```python
from build123d import *

# Parameters (mm, degrees)
F0_W      = 16
F0_H      = 16
F1_DEPTH  = 16
F2_R      = 2.54
F2_R_2    = 0.083649
F3_DEPTH  = 1.27
F3_FACE_R = 0.083649
F4_DEPTH  = 1.27
F5_R      = 2.54
F6_DEPTH  = 1.27
F7_DEPTH  = 1.27
F8_R      = 1.905
F8_R_2    = 1.900447
F9_DEPTH  = 1.27
F10_R     = 1.905
F11_DEPTH = 1.27
F12_R     = 1.872316
F12_R_2   = 1.905
F14_DEPTH = 1.27


with BuildPart() as f1:
    # F0 (on Front) → F1 (new body)
    with BuildSketch(Plane.XZ):
        with Locations((30.6324, 48.480009)):
            Rectangle(F0_W, F0_H)
    extrude(amount=-F1_DEPTH)

    # F2 (on face) → F3 (cut)
    with BuildSketch(Plane.XZ):
        with Locations((30.6324, 48.39636)):
            Circle(F2_R)
        with Locations((30.6324, 48.39636)):
            Circle(F2_R_2, mode=Mode.SUBTRACT)
    extrude(amount=-F3_DEPTH, mode=Mode.SUBTRACT)

    # F3_face (on face) → F4 (cut)
    with BuildSketch(Plane(origin=(30.6324, 0, 48.39636), x_dir=(1, 0, 0), z_dir=(0, -1, 0))):
        Circle(F3_FACE_R)
    extrude(amount=-F4_DEPTH, mode=Mode.SUBTRACT)

    # F5 (on face) → F6 (cut)
    with BuildSketch(Plane(origin=(22.6324, 0, 0), x_dir=(0, -1, 0), z_dir=(-1, 0, 0))):
        with Locations((-11.092744, 52.449955)):
            Circle(F5_R)
    extrude(amount=-F6_DEPTH, mode=Mode.SUBTRACT)

    # F5 (on face) → F7 (cut)
    with BuildSketch(Plane(origin=(22.6324, 0, 0), x_dir=(0, -1, 0), z_dir=(-1, 0, 0))):
        with Locations((-11.092744, 52.449955)):
            Circle(F5_R)
        with Locations((-5.08, 44.290009)):
            Circle(F5_R)
    extrude(amount=-F7_DEPTH, mode=Mode.SUBTRACT)

    # F8 (on face) → F9 (cut)
    with BuildSketch(Plane(origin=(0, 16, 0), x_dir=(-1, 0, 0), z_dir=(0, 1, 0))):
        with Locations((-34.8224, 52.924009)):
            Circle(F8_R)
        with Locations((-34.8224, 48.352009)):
            Circle(F8_R)
        with Locations((-34.8224, 43.780009)):
            Circle(F8_R)
        with Locations((-26.4424, 52.926009)):
            Circle(F8_R_2)
        with Locations((-26.4424, 43.782009)):
            Circle(F8_R)
        with Locations((-26.4424, 48.354009)):
            Circle(F8_R)
    extrude(amount=-F9_DEPTH, mode=Mode.SUBTRACT)

    # F10 (on face) → F11 (cut)
    with BuildSketch(Plane.YZ.offset(38.6324)):
        with Locations((8, 48.480009)):
            Circle(F10_R)
        with Locations((2.677711, 53.688009)):
            Circle(F10_R)
        with Locations((12.837711, 53.432009)):
            Circle(F10_R)
        with Locations((13.179603, 43.272009)):
            Circle(F10_R)
        with Locations((3.019603, 43.528009)):
            Circle(F10_R)
    extrude(amount=-F11_DEPTH, mode=Mode.SUBTRACT)

    # F12 (on face) → F14 (cut)
    with BuildSketch(Plane(origin=(0, 0, 40.480009), x_dir=(1, 0, 0), z_dir=(0, 0, -1))):
        with Locations((35.3324, -11.43)):
            Circle(F12_R)
        with Locations((30.5064, -7.72982)):
            Circle(F12_R_2)
        with Locations((26.4424, -3.360859)):
            Circle(F12_R_2)
    extrude(amount=-F14_DEPTH, mode=Mode.SUBTRACT)


solid = f1.part
```
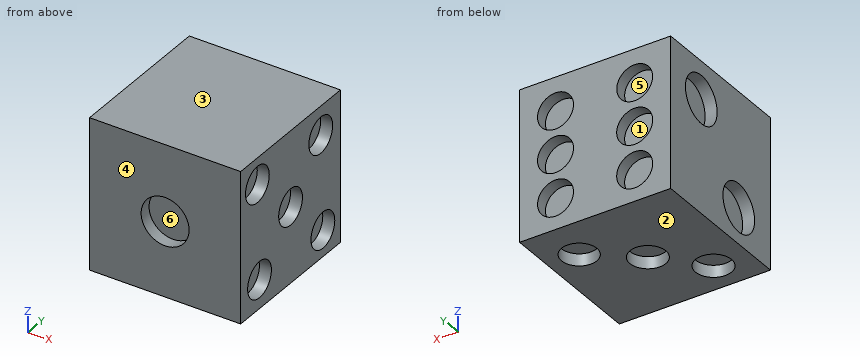
Read the model definition and answer for the solid it produces. Units are mm, in the model's axes. Face numbers are marked on the shaded views. A direction names the side the tool comes from. Give positions to 0.01 mm unless a question says otherwise; leave off trailing zeros. Order: outer loops, then holes, each group sorted by start corner. A loop starts at its lowest first (then second) coordinate and runs counter-clockwise, first axis right, second up.
(1) For the marked faces 4, 5 and 6, determine the directions among +Z, -Z, +X, -X, +Y, -Y from which every point of the face is accessible in a straight line to the end or side of a thin tool.
(2) Straight lines are drawn through the part: L1, parallel to X at y = 15, z = 48; L2, parallel to Z at x = 37.75, y = 8 (3 decimals); L3, parallel to Z at x = 27.75, y = 4.25. For each, find the intervals that lie inside material, in ascending order.
(3) Find section A-A (y = 4.25). Give the vertices of the cut face in (x, z).
(4) Given pin 1 (3 mm diameter, centred on y = 13, z = 53, fed in from +X); pin 2 (1.1 mm diameter, centred on y = 13.5, z = 44, fed in from +X); pin 3 (1.5 mm diameter, centred on y = 4, z = 43, fed in from -X); pin 4 (1.1 mm diameter, centred on x = 27, y = 3, fed in from -Z), each flat-ended and moving along its own axis, determine where each tip first touches the part or whether it passes through.
(5) Find section D-D (x = 30.5). Give the vertices of the cut face in (y, z), plus the area to 3 significant figures.
(6) Find section B-B (x = 34.75). Give the vertices of the cut face in (y, z).
(7) For a pull along Z with two mould halves and no side action, classify the marked faces 1, 2 and 3 as released by +Z, released by -Z, zero draft, split by the parting line, or undercut.
(8) Find section C-C (y = 8). Give the vertices of the cut face in (x, z) (3 decimals), plus the area to 3 significant figures.
Result sheet:
1. face 4: +Z, -Z, +X, -X, -Y
1. face 5: +Y
1. face 6: -Y
2. L1: x = 22.63 to 24.57, 28.31 to 32.95, 36.69 to 38.63
2. L2: z = 40.48 to 46.575, 50.385 to 56.48
2. L3: z = 41.75 to 56.48
3. outline: (22.63, 40.48) - (24.76, 40.48) - (24.76, 41.75) - (28.13, 41.75) - (28.13, 40.48) - (38.63, 40.48) - (38.63, 42.07) - (37.36, 42.07) - (37.36, 44.98) - (38.63, 44.98) - (38.63, 52.61) - (37.36, 52.61) - (37.36, 54.76) - (38.63, 54.76) - (38.63, 56.48) - (22.63, 56.48) - (22.63, 46.69) - (23.9, 46.69) - (23.9, 41.89) - (22.63, 41.89) - close
4. pin 1: stops at x = 38.63
4. pin 2: stops at x = 37.36
4. pin 3: stops at x = 23.9
4. pin 4: stops at z = 41.75
5. outline: (0, 40.48) - (5.82, 40.48) - (5.82, 41.75) - (9.63, 41.75) - (9.63, 40.48) - (16, 40.48) - (16, 56.48) - (0, 56.48) - (0, 50.93) - (1.27, 50.93) - (1.27, 45.86) - (0, 45.86) - close
5. area: 245 mm2
6. outline: (0, 40.48) - (9.65, 40.48) - (9.65, 41.75) - (13.21, 41.75) - (13.21, 40.48) - (16, 40.48) - (16, 41.88) - (14.73, 41.88) - (14.73, 45.68) - (16, 45.68) - (16, 46.45) - (14.73, 46.45) - (14.73, 50.26) - (16, 50.26) - (16, 51.02) - (14.73, 51.02) - (14.73, 54.83) - (16, 54.83) - (16, 56.48) - (0, 56.48) - close
7. face 1: undercut
7. face 2: released by -Z
7. face 3: released by +Z
8. outline: (22.632, 40.48) - (28.621, 40.48) - (28.621, 41.75) - (32.392, 41.75) - (32.392, 40.48) - (38.632, 40.48) - (38.632, 46.575) - (37.362, 46.575) - (37.362, 50.385) - (38.632, 50.385) - (38.632, 56.48) - (22.632, 56.48) - close
8. area: 246 mm2
